The figure shows three views and two pictorial views of one solid part (mm, origin at its lowest corner). Answer the questions. A direction names the side the tool comes from. Round coordinates to 2 decimals unless told otherwise and drop trailing zeros. Write each loop counter-clockwise with the first axis right and the second up, starting at its lowest first coordinate (ties: lowest second). Pieces come first, ordered by that corner, then holes.
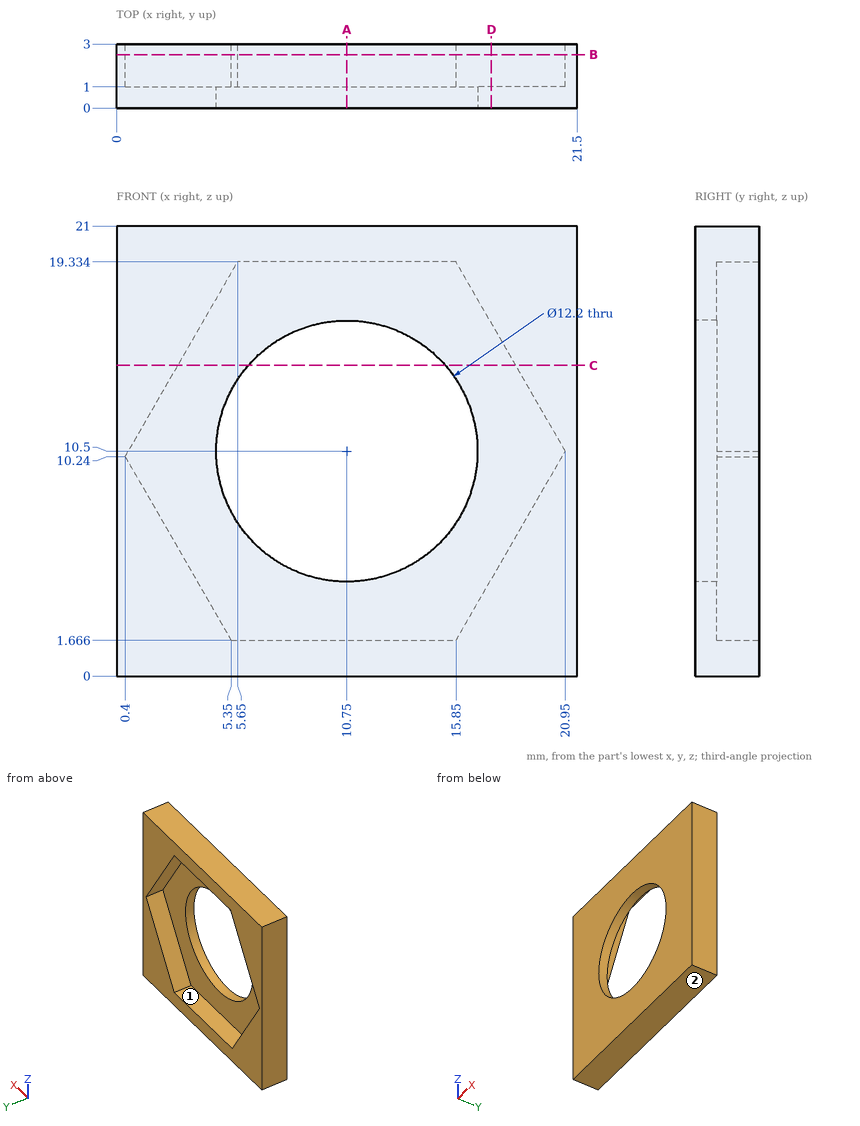
Q1. Straight lines are drawn through the part: probe 1 along Z at (x, y) = (10.75, 0.7); probe 2 along Z at (x, y) = (10.5, 1.8); probe 3 along X at (y, z) = (2.85, 4.75). For each, find the intervals that lie inside material, in ascending order.
Verdict:
probe 1: z = 0 to 4.4, 16.6 to 21
probe 2: z = 0 to 1.67, 19.33 to 21
probe 3: x = 0 to 3.57, 17.63 to 21.5
Q2. Section B-B (y = 2.5) is taken. Determine the outline of the cut face in (x, z).
Verdict:
outline: (0, 0) - (21.5, 0) - (21.5, 21) - (0, 21) - close; hole (0.4, 10.24) - (5.35, 1.67) - (15.85, 1.67) - (20.95, 10.5) - (15.85, 19.33) - (5.65, 19.33) - close
Q3. Section A-A (x = 10.75) is taken. Determine the outline of the cut face in (y, z).
Verdict:
outline: (0, 0) - (3, 0) - (3, 1.67) - (1, 1.67) - (1, 4.4) - (0, 4.4) - close; (0, 16.6) - (1, 16.6) - (1, 19.33) - (3, 19.33) - (3, 21) - (0, 21) - close
Q4. Which of the six approach directions +Z, -Z, +X, -X, +Y, -Y give full straight-line access (tool end or side, diameter ignored) to the marked faces 1 and 2?
Verdict:
face 1: +Y
face 2: -Z, +X, -X, +Y, -Y
Q5. Section C-C (z = 14.5) is taken. Determine the outline of the cut face in (x, y) (1 decimal).
Verdict:
outline: (0, 0) - (6.1, 0) - (6.1, 1) - (2.9, 1) - (2.9, 3) - (0, 3) - close; (15.4, 0) - (21.5, 0) - (21.5, 3) - (18.6, 3) - (18.6, 1) - (15.4, 1) - close
Q6. Section D-D (x = 17.5) is taken. Determine the outline of the cut face in (y, z) (1 decimal).
Verdict:
outline: (0, 0) - (3, 0) - (3, 4.5) - (1, 4.5) - (1, 16.5) - (3, 16.5) - (3, 21) - (0, 21) - close
